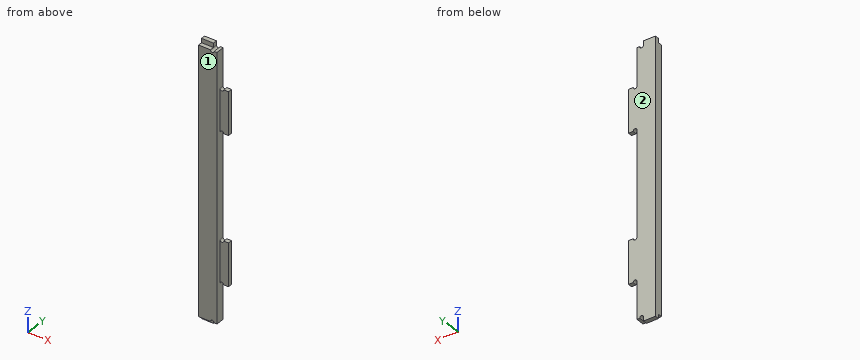
```python
from build123d import *

# Parameters (mm, degrees)
F1_DEPTH = 18
F0_W     = 25.45
F0_H     = 9
F2_DEPTH = 9


with BuildPart() as f1:
    # F0 (on Front) → F1 (new body)
    with BuildSketch(Plane.XZ):
        with BuildLine():
            Line((-27.599424, 185.439078), (-27.599424, 276.439078))
            Line((-27.599424, 276.439078), (-27.599424, 278.939078))
            Line((-27.599424, 278.939078), (-27.599424, 355.939078))
            Line((-27.599424, 355.939078), (-33.599424, 355.939078))
            ThreePointArc((-33.599424, 355.939078), (-37.599424, 351.939078), (-41.599424, 355.939078))
            Line((-41.599424, 355.939078), (-67.049424, 355.939078))
            Line((-67.049424, 355.939078), (-67.049424, -208.060922))
            Line((-67.049424, -208.060922), (-41.599424, -208.060922))
            ThreePointArc((-41.599424, -208.060922), (-37.599424, -204.060922), (-33.599424, -208.060922))
            Line((-33.599424, -208.060922), (-27.599424, -208.060922))
            Line((-27.599424, -208.060922), (-27.599424, -131.060922))
            Line((-27.599424, -131.060922), (-27.599424, -128.560922))
            Line((-27.599424, -128.560922), (-27.599424, -37.560922))
            Line((-27.599424, -37.560922), (-27.599424, -35.060922))
            Line((-27.599424, -35.060922), (-27.599424, 182.939078))
            Line((-27.599424, 182.939078), (-27.599424, 185.439078))
        make_face()
    extrude(amount=F1_DEPTH)

    # F0 (on Front) → F2 (join)
    with BuildSketch(Plane.XZ):
        with Locations((-54.324424, 360.439078)):
            Rectangle(F0_W, F0_H)
        with BuildLine():
            ThreePointArc((-19.599424, 276.439078), (-23.599424, 272.439078), (-27.599424, 276.439078))
            Line((-27.599424, 276.439078), (-27.599424, 185.439078))
            ThreePointArc((-27.599424, 185.439078), (-23.599424, 189.439078), (-19.599424, 185.439078))
            Line((-19.599424, 185.439078), (-9.599424, 185.439078))
            Line((-9.599424, 185.439078), (-9.599424, 276.439078))
            Line((-9.599424, 276.439078), (-19.599424, 276.439078))
        make_face()
        with BuildLine():
            ThreePointArc((-19.599424, -37.560922), (-23.599424, -41.560922), (-27.599424, -37.560922))
            Line((-27.599424, -37.560922), (-27.599424, -128.560922))
            ThreePointArc((-27.599424, -128.560922), (-23.599424, -124.560922), (-19.599424, -128.560922))
            Line((-19.599424, -128.560922), (-9.599424, -128.560922))
            Line((-9.599424, -128.560922), (-9.599424, -37.560922))
            Line((-9.599424, -37.560922), (-19.599424, -37.560922))
        make_face()
        with Locations((-54.324424, -212.560922)):
            Rectangle(F0_W, F0_H)
    extrude(amount=F2_DEPTH)


solid = f1.part
```
The model under review builds one solid part; all positions refer to its coordinate system, in mm. Face numbers are marked on the shaded views. Round coordinates to 2 decimals unless told otherwise and drop trailing zeros. Write each loop counter-clockwise with the first axis right and the second up, starting at its lowest first coordinate (ties: lowest second). Pieces come first, ordered by that corner, then holes.
(1) We need section A-A on y = -5. Give the boundary of the cut face in (x, z), and give its area (3 significant figures).
(2) Mouldability with a two-part tool opening along Y and no side actions: class the marked faces 1 and 2 as +Y half, -Y half, draft (parallel to the pull), parting line (faces both ways), or undercut.
(3) Wall thickness on L1, parallel to X at y = -13.5, z = 3; L2, parallel to Z at x = -15, y = -2.5; L3, parallel to Z at x = -64.5, y = -9.75: over which ranges is each line inside the solid? List them lowest first.
(4) We need section B-B on x = -52. Give the boundary of the cut face in (y, z), and give its area (3 significant figures).
(5) Insertion check: pin 1 (7 mm diameter, centred on x = -12.5, y = -5.5, fed in from +Z); pin 2 (14.5 mm diameter, centred on x = -18, z = -77.5, fed in from -Y); pin 3 (10 mm diameter, centred on x = -55, z = 123, fed in from +Y); pin 4 (1.5 mm diameter, centred on y = -14, z = 48.5, fed in from +X). Each pin has a flat end and moves straight along its axis. Give the tip position at first contact, or say it passes through.
(6) We need section C-C on z = -76.5. Give the boundary of the cut face in (x, y).
Findings below:
1. outline: (-67.05, -217.06) - (-41.6, -217.06) - (-41.6, -208.06) arc R4 cw to (-33.6, -208.06) - (-27.6, -208.06) - (-27.6, -128.56) arc R4 cw to (-19.6, -128.56) - (-9.6, -128.56) - (-9.6, -37.56) - (-19.6, -37.56) arc R4 cw to (-27.6, -37.56) - (-27.6, 185.44) arc R4 cw to (-19.6, 185.44) - (-9.6, 185.44) - (-9.6, 276.44) - (-19.6, 276.44) arc R4 cw to (-27.6, 276.44) - (-27.6, 355.94) - (-33.6, 355.94) arc R4 cw to (-41.6, 355.94) - (-41.6, 364.94) - (-67.05, 364.94) - close
1. area: 25,800 mm2
2. face 1: -Y half
2. face 2: +Y half
3. L1: x = -67.05 to -27.6
3. L2: z = -128.56 to -37.56, 185.44 to 276.44
3. L3: z = -208.06 to 355.94
4. outline: (-18, -208.06) - (-9, -208.06) - (-9, -217.06) - (0, -217.06) - (0, 364.94) - (-9, 364.94) - (-9, 355.94) - (-18, 355.94) - close
4. area: 10,300 mm2
5. pin 1: stops at z = 276.44
5. pin 2: stops at y = -9
5. pin 3: stops at y = 0
5. pin 4: stops at x = -27.6
6. outline: (-67.05, -18) - (-27.6, -18) - (-27.6, -9) - (-9.6, -9) - (-9.6, 0) - (-67.05, 0) - close
